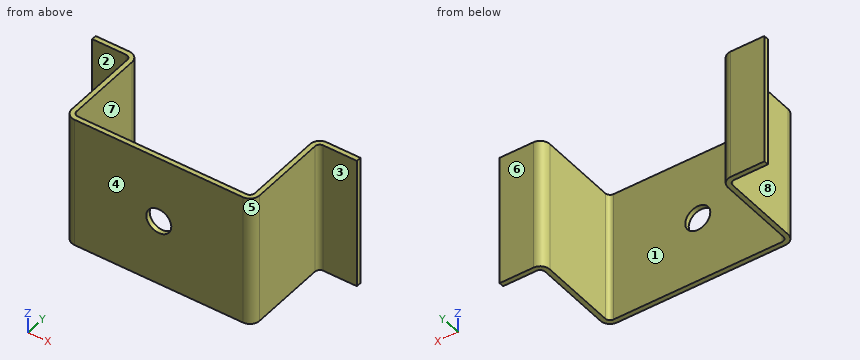
from build123d import *

# Parameters (mm, degrees)
SKETCH1_W                      = 78
SKETCH1_H                      = 2
BASE_FLANGE1_DEPTH             = 27.5
EDGE_FLANGE1_STRIP_W           = 12
EDGE_FLANGE1_STRIP_H           = 2
EDGE_FLANGE1_STRIP_CUT_DEPTH   = 55
EDGE_FLANGE1_STRIP_2_W         = 12
EDGE_FLANGE1_STRIP_2_H         = 2
EDGE_FLANGE1_STRIP_CUT_2_DEPTH = 55
EDGE_FLANGE1_DEPTH             = 55
EDGE_FLANGE1_BEND_DEPTH        = 55
EDGE_FLANGE2_STRIP_W           = 12
EDGE_FLANGE2_STRIP_H           = 2
EDGE_FLANGE2_STRIP_CUT_DEPTH   = 55
EDGE_FLANGE2_STRIP_2_W         = 12
EDGE_FLANGE2_STRIP_2_H         = 2
EDGE_FLANGE2_STRIP_CUT_2_DEPTH = 55
EDGE_FLANGE2_DEPTH             = 55
EDGE_FLANGE2_BEND_DEPTH        = 55
SKETCH18_R                     = 5.2
CUT_EXTRUDE1_DEPTH             = 10


# Sheet-metal steps are written as plain solids
with BuildPart() as part:
    # Sketch1 → Base-Flange1 (new, symmetric)
    with BuildSketch(Plane.XY):
        with Locations((0, 1)):
            Rectangle(SKETCH1_W, SKETCH1_H)
    extrude(amount=BASE_FLANGE1_DEPTH, both=True)

    # Edge-Flange1 strip (across the edge) → Edge-Flange1 strip cut (cut)
    with BuildSketch(Plane(origin=(-39, 2, -27.5), x_dir=(1, 0, 0), z_dir=(0, 0, 1))):
        with Locations((-2, -1)):
            Rectangle(EDGE_FLANGE1_STRIP_W, EDGE_FLANGE1_STRIP_H)
    extrude(amount=EDGE_FLANGE1_STRIP_CUT_DEPTH, mode=Mode.SUBTRACT)

    # Edge-Flange1 strip 2 (across the edge) → Edge-Flange1 strip cut 2 (cut)
    with BuildSketch(Plane(origin=(39, 2, 27.5), x_dir=(-1, 0, 0), z_dir=(0, 0, -1))):
        with Locations((-2, -1)):
            Rectangle(EDGE_FLANGE1_STRIP_2_W, EDGE_FLANGE1_STRIP_2_H)
    extrude(amount=EDGE_FLANGE1_STRIP_CUT_2_DEPTH, mode=Mode.SUBTRACT)

    # Edge-Flange1 section (across the edge) → Edge-Flange1 (add)
    with BuildSketch(Plane(origin=(-39, 2, -27.5), x_dir=(1, 0, 0), z_dir=(0, 0, 1))):
        with BuildLine():
            Line((0, 2), (0, 38))
            Line((0, 38), (2, 38))
            Line((2, 38), (2, 2))
            ThreePointArc((2, 2), (2.585786438, 0.585786438), (4, 0))
            Line((4, 0), (4, -2))
            ThreePointArc((4, -2), (1.171572875, -0.828427125), (0, 2))
        make_face()
    extrude(amount=EDGE_FLANGE1_DEPTH)

    # Edge-Flange1 section 2 (across the edge) → Edge-Flange1 bend (add)
    with BuildSketch(Plane(origin=(39, 2, 27.5), x_dir=(-1, 0, 0), z_dir=(0, 0, -1))):
        with BuildLine():
            Line((0, 2), (0, 38))
            Line((0, 38), (2, 38))
            Line((2, 38), (2, 2))
            ThreePointArc((2, 2), (2.585786438, 0.585786438), (4, 0))
            Line((4, 0), (4, -2))
            ThreePointArc((4, -2), (1.171572875, -0.828427125), (0, 2))
        make_face()
    extrude(amount=EDGE_FLANGE1_BEND_DEPTH)

    # Edge-Flange2 strip (across the edge) → Edge-Flange2 strip cut (cut)
    with BuildSketch(Plane(origin=(39, 40, -27.5), x_dir=(0, -1, 0), z_dir=(0, 0, 1))):
        with Locations((-2, -1)):
            Rectangle(EDGE_FLANGE2_STRIP_W, EDGE_FLANGE2_STRIP_H)
    extrude(amount=EDGE_FLANGE2_STRIP_CUT_DEPTH, mode=Mode.SUBTRACT)

    # Edge-Flange2 strip 2 (across the edge) → Edge-Flange2 strip cut 2 (cut)
    with BuildSketch(Plane(origin=(-39, 40, 27.5), x_dir=(0, -1, 0), z_dir=(0, 0, -1))):
        with Locations((-2, -1)):
            Rectangle(EDGE_FLANGE2_STRIP_2_W, EDGE_FLANGE2_STRIP_2_H)
    extrude(amount=EDGE_FLANGE2_STRIP_CUT_2_DEPTH, mode=Mode.SUBTRACT)

    # Edge-Flange2 section (across the edge) → Edge-Flange2 (add)
    with BuildSketch(Plane(origin=(39, 40, -27.5), x_dir=(0, -1, 0), z_dir=(0, 0, 1))):
        with BuildLine():
            Line((0, 2), (0, 16))
            Line((0, 16), (2, 16))
            Line((2, 16), (2, 2))
            ThreePointArc((2, 2), (2.585786438, 0.585786438), (4, 0))
            Line((4, 0), (4, -2))
            ThreePointArc((4, -2), (1.171572875, -0.828427125), (0, 2))
        make_face()
    extrude(amount=EDGE_FLANGE2_DEPTH)

    # Edge-Flange2 section 2 (across the edge) → Edge-Flange2 bend (add)
    with BuildSketch(Plane(origin=(-39, 40, 27.5), x_dir=(0, -1, 0), z_dir=(0, 0, -1))):
        with BuildLine():
            Line((0, 2), (0, 16))
            Line((0, 16), (2, 16))
            Line((2, 16), (2, 2))
            ThreePointArc((2, 2), (2.585786438, 0.585786438), (4, 0))
            Line((4, 0), (4, -2))
            ThreePointArc((4, -2), (1.171572875, -0.828427125), (0, 2))
        make_face()
    extrude(amount=EDGE_FLANGE2_BEND_DEPTH)

    # Sketch18 → Cut-Extrude1 (cut)
    with BuildSketch(Plane(origin=(0, 2, 0), x_dir=(1, 0, 0), z_dir=(0, 1, 0))):
        with Locations(Location((0, 0, 0), (0, 0, 270))):
            Circle(SKETCH18_R)
    extrude(amount=-CUT_EXTRUDE1_DEPTH, mode=Mode.SUBTRACT)


solid = part.part
Check sheet for the modelled part. Datum: model origin and axes. Units: mm. Face numbers are marked on the shaded views. A direction names the side the tool comes from. Round coordinates to 2 decimals unless told otherwise and drop trailing zeros. Write each loop counter-clockwise with the first axis right and the second up, starting at its lowest first coordinate (ties: lowest second). Pieces come first, ordered by that corner, then holes. Notation, with made-up numbers: (72, -1) - (120, -1) arc R26 cw to (120, 22) - close; hole circle Ø2 at (-40, 40.25). An arc over 180 degrees is marked (long way). Return JSON: item names as keys, results as strings.
Q1. Cross-section at C-C (x = 0). Record the boundary of the cut face in (y, z).
Returned:
{"outline": "(0, -27.5) - (2, -27.5) - (2, -5.2) - (0, -5.2) - close; (0, 5.2) - (2, 5.2) - (2, 27.5) - (0, 27.5) - close"}
Q2. Cross-section at A-A (y = 24). Record the boundary of the cut face in (x, z), then the cut area to 3 significant figures.
Returned:
{"outline": "(-39, -27.5) - (-37, -27.5) - (-37, 27.5) - (-39, 27.5) - close; (37, -27.5) - (39, -27.5) - (39, 27.5) - (37, 27.5) - close", "area": "220 mm²"}
Q3. Access from +Z, -Z, +X, -X, +Y, -Y to the whole of each face (thin tool, end or side, straight path). Record for the marked faces 1, 2, 3 and 4.
Returned:
{"face 1": "+Z, -Z, +Y", "face 2": "+Z, -Z, -X, -Y", "face 3": "+Z, -Z, +X, -Y", "face 4": "+Z, -Z, +X, -X, -Y"}
Q4. Depth check by flat-ended pin: P1, Ø7, axis at x = 46, z = -6.5, coming from the -Y side; P2, Ø3, axis at y = 9.5, z = 16.5, coming from the +X side; P3, Ø10, axis at y = 23.5, z = -16, coming from the -X side. Enter the tip coordinate at first touch or a pass-through.
Returned:
{"P1": "stops at y = 38", "P2": "stops at x = 39", "P3": "stops at x = -39"}
Q5. Draft check along X on the marked faces 5, 6, 7 and 8. Enter one of: released by +X, released by -X, zero draft, split by the parting line, or undercut.
Returned:
{"face 5": "released by +X", "face 6": "zero draft", "face 7": "undercut", "face 8": "released by -X"}
Q6. Cross-section at D-D (z = -14). Record the boundary of the cut face in (x, y), then the cut area to 3 significant figures.
Returned:
{"outline": "(-55, 38) - (-41, 38) arc R2 cw to (-39, 36) - (-39, 4) arc R4 ccw to (-35, 0) - (35, 0) arc R4 ccw to (39, 4) - (39, 36) arc R2 cw to (41, 38) - (55, 38) - (55, 40) - (41, 40) arc R4 ccw to (37, 36) - (37, 4) arc R2 cw to (35, 2) - (-35, 2) arc R2 cw to (-37, 4) - (-37, 36) arc R4 ccw to (-41, 40) - (-55, 40) - close", "area": "362 mm²"}
Q7. Cross-section at B-B (z = 0). Record the boundary of the cut face in (x, y).
Returned:
{"outline": "(-55, 38) - (-41, 38) arc R2 cw to (-39, 36) - (-39, 4) arc R4 ccw to (-35, 0) - (-5.2, 0) - (-5.2, 2) - (-35, 2) arc R2 cw to (-37, 4) - (-37, 36) arc R4 ccw to (-41, 40) - (-55, 40) - close; (5.2, 0) - (35, 0) arc R4 ccw to (39, 4) - (39, 36) arc R2 cw to (41, 38) - (55, 38) - (55, 40) - (41, 40) arc R4 ccw to (37, 36) - (37, 4) arc R2 cw to (35, 2) - (5.2, 2) - close"}
Q8. Scan lines: L1, parallel to X at y = 7, z = 16; L2, parallel to Y at x = -16, z = -14; L3, parallel to X at y = 1, z = 0. Record each from-to range of solid material in increasing order. Write a range as from..to.
Returned:
{"L1": "x = -39..-37, 37..39", "L2": "y = 0..2", "L3": "x = -37.65..-5.2, 5.2..37.65"}
